Geometry: see drawing. Coordinates: mm, zero at the bounding-box minimum. A direction names the side the tool comes from. Give positions to 0.01 mm unless a question says otherwise; leave off trailing zeros. Loops run counter-clockwise (first coordinate to the right, second up) from the corner with the lowest first, then second, coordinate; pieces in that order, holes last. Notation, with made-up numbers: (51.25, -25) - (70.25, -25) arc R6 cw to (70.25, -21) - close; hole circle Ø10 at (30, -29). An arc over 180 degrees is marked (long way). One line per question, with ' | ' between items. Start each with the question number.
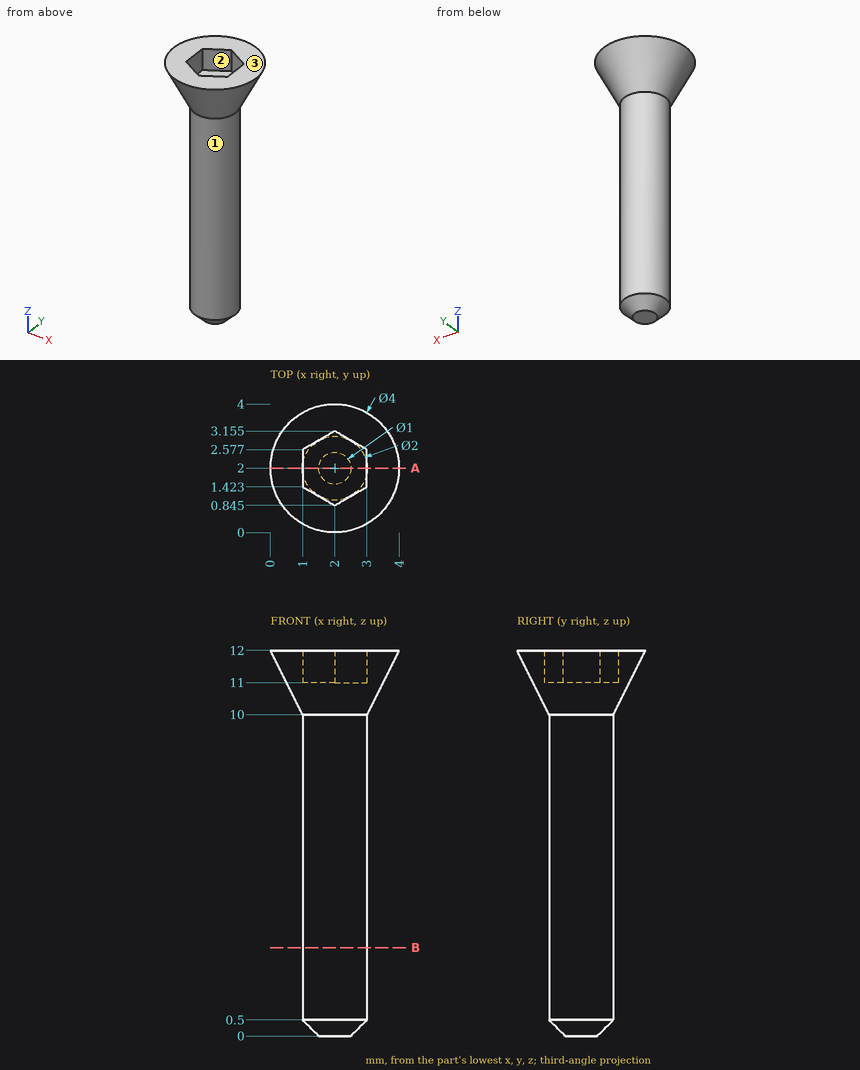
Q1. Access query for the marked faces 1, 2 and 3. Directions: +Z, -Z, +X, -X, +Y, -Y. A direction counts if a zero-diameter tool reaches every point of the face in a straight line with its end or side. Return the directions, or none.
Q2. Section A-A, the plane y = 2. Output: boundary loops of the cut face in (x, z).
Q3. First-contact query: pin 1 (1 mm diameter, centred on x = 1.5, z = 2.5, fed in from +Y); pin 2 (1.5 mm diameter, centred on x = 1.5, z = 10.5, fed in from -Y) (1 decimal); pin 3 (0.5 mm diameter, centred on y = 1.5, z = 11.5, fed in from +X). Flat tips, straight axial feed; report the tip coordinate or a pass-through.
Q4. Section B-B, the plane z = 2.75. Output: boundary loops of the cut face in (x, y).
Q5. Line query: L1, parallel to Y at x = 1.95, z = 8; L2, parallel to Z at x = 3, y = 3.4; L3, parallel to X at y = 2.2, z = 2. Output: solid intervals per line, ascending. Write a range as from..to.
Solved:
1) face 1: -Z | face 2: +Z | face 3: +Z, +X, -X, +Y, -Y
2) outline: (0, 12) - (1, 10) - (1, 0.5) - (1.5, 0) - (2.5, 0) - (3, 0.5) - (3, 10) - (4, 12) - (3, 12) - (3, 11) - (1, 11) - (1, 12) - close
3) pin 1: stops at y = 3 | pin 2: stops at y = 0.4 | pin 3: stops at x = 3.82
4) outline: circle Ø2 at (2, 2)
5) L1: y = 1..3 | L2: z = 11.44..12 | L3: x = 1.02..2.98
